from build123d import *

# Parameters (mm, degrees)
SKETCH1_W           = 10
SKETCH1_H           = 15.7
SKETCH1_R           = 1.6
BOSS_EXTRUDE1_DEPTH = 1.5
SKETCH2_W           = 10
SKETCH2_H           = 8.7
BOSS_EXTRUDE2_DEPTH = 3
SKETCH4_W           = 1.3
SKETCH4_H           = 0.8
BOSS_EXTRUDE3_DEPTH = 6.8
SKETCH5_R           = 0.4
BOSS_EXTRUDE4_DEPTH = 2


with BuildPart() as part:
    # Sketch1 → Boss-Extrude1 (new body)
    with BuildSketch(Plane.XY):
        with Locations((0, -4.35)):
            Rectangle(SKETCH1_W, SKETCH1_H)
        Circle(SKETCH1_R, mode=Mode.SUBTRACT)
    extrude(amount=BOSS_EXTRUDE1_DEPTH)

    # Sketch2 → Boss-Extrude2 (add)
    with BuildSketch(Plane.XY.offset(1.5)):
        with Locations((0, -7.85)):
            Rectangle(SKETCH2_W, SKETCH2_H)
    extrude(amount=BOSS_EXTRUDE2_DEPTH)

    # Sketch4 → Boss-Extrude3 (add)
    with BuildSketch(Plane.XZ.offset(12.2)):
        with Locations((-3.25, 2.25)):
            Rectangle(SKETCH4_W, SKETCH4_H)
        with Locations((-1.625, 2.25)):
            Rectangle(SKETCH4_W, SKETCH4_H)
        with Locations((0, 2.25)):
            Rectangle(SKETCH4_W, SKETCH4_H)
        with Locations((1.625, 2.25)):
            Rectangle(SKETCH4_W, SKETCH4_H)
        with Locations((3.25, 2.25)):
            Rectangle(SKETCH4_W, SKETCH4_H)
    extrude(amount=BOSS_EXTRUDE3_DEPTH)

    # Sketch5 → Boss-Extrude4 (add)
    with BuildSketch(Plane.XZ.offset(19)):
        with Locations(Location((-3.25, 2.25, 0), (0, 0, 270))):
            Circle(SKETCH5_R)
        with Locations(Location((-1.625, 2.25, 0), (0, 0, 270))):
            Circle(SKETCH5_R)
        with Locations(Location((0, 2.25, 0), (0, 0, 270))):
            Circle(SKETCH5_R)
        with Locations(Location((1.625, 2.25, 0), (0, 0, 270))):
            Circle(SKETCH5_R)
        with Locations(Location((3.25, 2.25, 0), (0, 0, 270))):
            Circle(SKETCH5_R)
    extrude(amount=BOSS_EXTRUDE4_DEPTH)


solid = part.part
For this review, take the finished solid that the model builds, in its own axes (mm). A direction names the side the tool comes from. Give positions to 0.01 mm unless a question says otherwise; leave off trailing zeros. Order: outer loops, then holes, each group sorted by start corner. A loop starts at its lowest first (then second) coordinate and runs counter-clockwise, first axis right, second up. Notation, with made-up numbers: M -18.75,77 L 20.25,77 A15 cw 20.25,96 Z; hole C -17,80 d7. An arc over 180 degrees is marked long. Answer in a Markdown table with one row per item. Add a question column.
(1) Mouldability with a two-part tool opening along Y and no side actions: class faces 5 (the face through (0, 3.5, 1)), 6 (the face through (2, -16, 2.65)), 7 (the face through (-1.27, -0.97, 0.74)) as +Y half, -Y half, draft (parallel to the pull), parting line (faces both ways), or undercut.
(2) Consider section A-A on y = 0. State the section outline as (x, z) points.
(3) Wall thickness on probe 1 along X at (y, z) = (-18.5, 2.6) (3 decimals); probe 2 along Y at (x, z) = (0, 1.15); probe 3 along Y at (x, z) = (-3.5, 4.3): over which ranges is each line inside the solid? List them lowest first. Write a range as [from, to].
(4) For faces 1 (the face through (0, 2, 1.5)), 2 (the face through (-2, -16, 1.85)), 3 (the face through (-3, -16, 2.65)), 4 (the face through (0, -8, 4.5)), list the 3-axis set-ups (+Z, -Z, +X, -X, +Y, -Y) from which the entire face can be reached by the end or side of a thin tool; tool diameter is ignored.
(5) Consider section B-B on z = 4. State the section outline as (x, y) points, and give its area (3 significant figures).
(6) For pin 1 (3 mm diameter, centred on x = 1.5, y = -7, fed in from -Z); pin 2 (0.6 mm diameter, centred on y = -17, z = 2.5, fed in from +X); pin 3 (2 mm diameter, centred on x = 1.5, z = 3.5, fed in from +Y); pin 4 (1.4 mm diameter, centred on x = 3, y = -15, fed in from +Z), all flat-tipped, find the tip position at first contact; note any pin that passes through.
Evaluation:
| question | item | result |
|---|---|---|
| 1 | face 5 | +Y half |
| 1 | face 6 | draft |
| 1 | face 7 | undercut |
| 2 | outline | M -5,0 L -1.6,0 L -1.6,1.5 L -5,1.5 Z; M 1.6,0 L 5,0 L 5,1.5 L 1.6,1.5 Z |
| 3 | probe 1 | x = [-3.9, -2.6], [-2.275, -0.975], [-0.65, 0.65], [0.975, 2.275], [2.6, 3.9] |
| 3 | probe 2 | y = [-12.2, -1.6], [1.6, 3.5] |
| 3 | probe 3 | y = [-12.2, -3.5] |
| 4 | face 1 | +Z, +X, -X, +Y |
| 4 | face 2 | -Z, +X, -X, -Y |
| 4 | face 3 | +Z, +X, -X, -Y |
| 4 | face 4 | +Z, +X, -X, +Y, -Y |
| 5 | outline | M -5,-12.2 L 5,-12.2 L 5,-3.5 L -5,-3.5 Z |
| 5 | area | 87.0 mm^2 |
| 6 | pin 1 | stops at z = 0 |
| 6 | pin 2 | stops at x = 3.9 |
| 6 | pin 3 | stops at y = -3.5 |
| 6 | pin 4 | stops at z = 2.65 |
